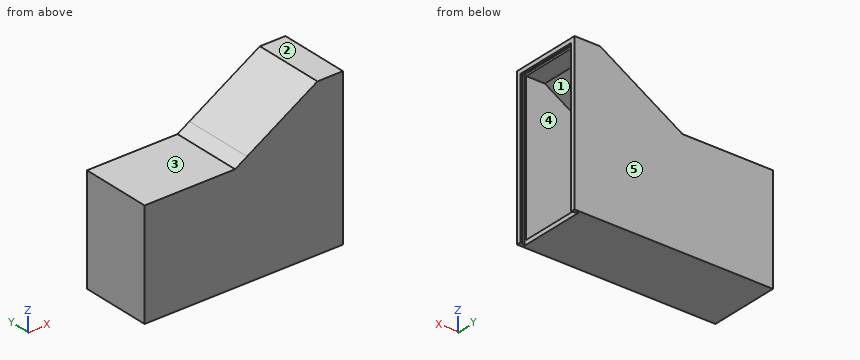
```python
from build123d import *

# Parameters (mm, degrees)
BOSS_EXTRUDE1_DEPTH = 25
BOSS_EXTRUDE2_DEPTH = 3
SKETCH5_W           = 3
SKETCH5_H           = 22
CUT_EXTRUDE1_DEPTH  = 1.5
SKETCH6_W           = 3
SKETCH6_H           = 107.5
CUT_EXTRUDE2_DEPTH  = 1.5
BOSS_EXTRUDE4_DEPTH = 23.5
BOSS_EXTRUDE5_DEPTH = 109


with BuildPart() as part:
    # PCB → Boss-Extrude1 (new body)
    with BuildSketch(Plane(origin=(0, 0, 0), x_dir=(1, 0, 0), z_dir=(0, 1, 0))):
        Polygon((118.862351474, -102.5), (71.5, -74.284131037), (71.5, -68), (-0.5, -68), (-0.5, 0.5), (132, 0.5), (132, 3.5), (-3.5, 3.5), (-3.5, -71), (60.125746031, -71), (68.5, -75.988917258), (118.036460317, -105.5), (135, -105.5), (136, -105.5), (136, -102.5), (132, -102.5), align=None)
    boss_extrude1 = extrude(amount=BOSS_EXTRUDE1_DEPTH)

    # Sketch4 → Boss-Extrude2 (add)
    with BuildSketch(Plane(origin=(0, 25, 0), x_dir=(1, 0, 0), z_dir=(0, 1, 0))):
        Polygon((118.862351474, -102.5), (136, -102.5), (136, 3.5), (132, 3.5), (132, 0.5), (-0.5, 0.5), (-0.5, -68), (71.5, -68), (71.5, -74.284131037), align=None)
    boss_extrude2 = extrude(amount=-BOSS_EXTRUDE2_DEPTH)

    # Sketch5 → Cut-Extrude1 (cut)
    with BuildSketch(Plane(origin=(0, 0, 102.5), x_dir=(-1, 0, 0), z_dir=(0, 0, -1))):
        with Locations((-133.5, 11)):
            Rectangle(SKETCH5_W, SKETCH5_H)
    cut_extrude1 = extrude(amount=-CUT_EXTRUDE1_DEPTH, mode=Mode.SUBTRACT)

    # Sketch6 → Cut-Extrude2 (cut)
    with BuildSketch(Plane.XZ.offset(-22)):
        with Locations((133.5, 50.25)):
            Rectangle(SKETCH6_W, SKETCH6_H)
    cut_extrude2 = extrude(amount=-CUT_EXTRUDE2_DEPTH, mode=Mode.SUBTRACT)

    # Sketch7 → Boss-Extrude4 (add)
    with BuildSketch(Plane.XZ.offset(-23.5)):
        Polygon((135, 102.5), (132, 104), (135, 104), align=None)
    boss_extrude4 = extrude(amount=BOSS_EXTRUDE4_DEPTH)

    # Sketch8 → Boss-Extrude5 (add)
    with BuildSketch(Plane.XY.offset(105.5)):
        Polygon((135, 22), (132, 23.5), (135, 23.5), align=None)
    boss_extrude5 = extrude(amount=-BOSS_EXTRUDE5_DEPTH)

    # Mirror2: Boss-Extrude1, Boss-Extrude2, Cut-Extrude1, Cut-Extrude2, Boss-Extrude4, Boss-Extrude5 across plane
    add(boss_extrude1.mirror(Plane.ZX))
    add(boss_extrude2.mirror(Plane.ZX))
    add(cut_extrude1.mirror(Plane.ZX), mode=Mode.SUBTRACT)
    add(cut_extrude2.mirror(Plane.ZX), mode=Mode.SUBTRACT)
    add(boss_extrude4.mirror(Plane.ZX))
    add(boss_extrude5.mirror(Plane.ZX))


solid = part.part
```
The listing builds one solid part. Answer for the finished solid, in the listing's coordinates (mm). Face numbers are marked on the shaded views. A direction names the side the tool comes from. Give positions to 0.01 mm unless a question says otherwise; leave off trailing zeros. Loops run counter-clockwise (first coordinate to the right, second up) from the corner with the lowest first, then second, coordinate; pieces in that order, holes last. Notation, with made-up numbers: (12, 31.25) - (24, 31.25) arc R18 ccw to (24, 66.25) - close; hole circle Ø11 at (-26.75, 47). An arc over 180 degrees is marked (long way). Return JSON: item names as keys, results as strings. Group by question number.
1. Straight lines are drawn through the part: line 1 (Y direction, x = 44, z = 52); line 2 (Z direction, x = 12, y = -21.5); line 3 (Z direction, x = 124, y = 11). For each, find the intervals that lie inside material, in ascending order. Write a range as [from, to].
2. Given pin 1 Ø0.5 at (x, y) = (135.5, -10.5) entering from -Z; pin 2 Ø7 at (y, z) = (-6.5, 72.5) entering from +X; pin 3 Ø1 at (y, z) = (-13.5, 81) entering from -X, each flat-ended and moving along its own axis, determine where each tip first touches the part or whether it passes through.
3. Find section D-D (z = 78). Write down the section's boundary in (x, y), then the cut area to 3 significant figures.
4. Find section A-A (x = 11.5). Write down the section's boundary in (y, z), then the cut area to 3 significant figures.
5. Determine the mould class of the marked faces 3, 4 and 5 for opening direction Z: pulls with the +Z half, pulls with the -Z half, needs draft (parallel to the pull), parting line crosses it, or undercut.
6. Find section B-B (z = 38). Write down the section's boundary in (x, y).
7. Which of the six approach directions +Z, -Z, +X, -X, +Y, -Y give full straight-line access (tool end or side, diameter ignored) to the marked faces 1 and 2?
8. Find section C-C (y = 1). Write down the section's boundary in (x, z).
Verdict:
{
 "1": {"line 1": "y = [-25, -22], [22, 25]", "line 2": "z = [-3.5, -0.5], [68, 71]", "line 3": "z = [-3.5, -0.5], [102.5, 105.5]"},
 "2": {"pin 1": "stops at z = 102.5", "pin 2": "stops at x = 74.38", "pin 3": "stops at x = 76.07"},
 "3": {"outline": "(71.88, -25) - (136, -25) - (136, -22) - (135, -22) - (132, -23.5) - (132, -22) - (77.74, -22) - (77.74, 22) - (132, 22) - (132, 23.5) - (135, 22) - (136, 22) - (136, 25) - (71.88, 25) - close", "area": "638 mm^2"},
 "4": {"outline": "(-25, -3.5) - (25, -3.5) - (25, 71) - (-25, 71) - close; hole (-22, -0.5) - (22, -0.5) - (22, 68) - (-22, 68) - close", "area": "711 mm^2"},
 "5": {"face 3": "pulls with the +Z half", "face 4": "undercut", "face 5": "needs draft"},
 "6": {"outline": "(-3.5, -25) - (136, -25) - (136, -22) - (135, -22) - (132, -23.5) - (132, -22) - (-0.5, -22) - (-0.5, 22) - (132, 22) - (132, 23.5) - (135, 22) - (136, 22) - (136, 25) - (-3.5, 25) - close"},
 "7": {"face 1": "+X", "face 2": "+Z, +X, -X, +Y, -Y"},
 "8": {"outline": "(-3.5, -3.5) - (132, -3.5) - (132, -0.5) - (-0.5, -0.5) - (-0.5, 68) - (71.5, 68) - (71.5, 74.28) - (118.86, 102.5) - (132, 102.5) - (132, 104) - (135, 102.5) - (136, 102.5) - (136, 105.5) - (118.04, 105.5) - (60.13, 71) - (-3.5, 71) - close"}
}
